Verification items for this drawing (mm, ordinates from the low corner). A direction names the side the tool comes from. Round coordinates to 2 decimals unless told otherwise and drop trailing zeros. Loops run counter-clockwise (first coordinate to the right, second up) from the corner with the lowest first, then second, coordinate; pieces in that order, holes last. Notation, with made-up numbers: M 77.5,59 L 89.5,59 A31 ccw 89.5,88 Z; hole C 77.5,-17 d3. An arc over 180 degrees is marked long. Use one line per item in the form item = value. Start each with the question number.
1. Cross-section at B-B (z = 46). Record the boundary of the cut face in (x, y), then the cut area to 3 significant figures.
2. Set-up check for the marked faces 1 and 2: record each of +Z, -Z, +X, -X, +Y, -Y from which the full face is reachable in a straight line by a thin tool's end or side.
3. Cross-section at A-A (x = 25). Record the boundary of the cut face in (y, z), then the cut area to 3 significant figures.
4. Go/stop test with flat-tipped pins: pin 1 (6 mm diameter, centred on x = 5, z = 43.5, fed in from -Y); pin 2 (1 mm diameter, centred on x = 25, y = 18.5, fed in from +Z); pin 3 (2 mm diameter, centred on x = 42.5, z = 20.5, fed in from +Y). Record where each tip stops, or that it passes through.
5. Material ranges on line 1 (Z direction, x = 35, y = 23); line 2 (Z direction, x = 38.5, y = 8), recorded low to high.
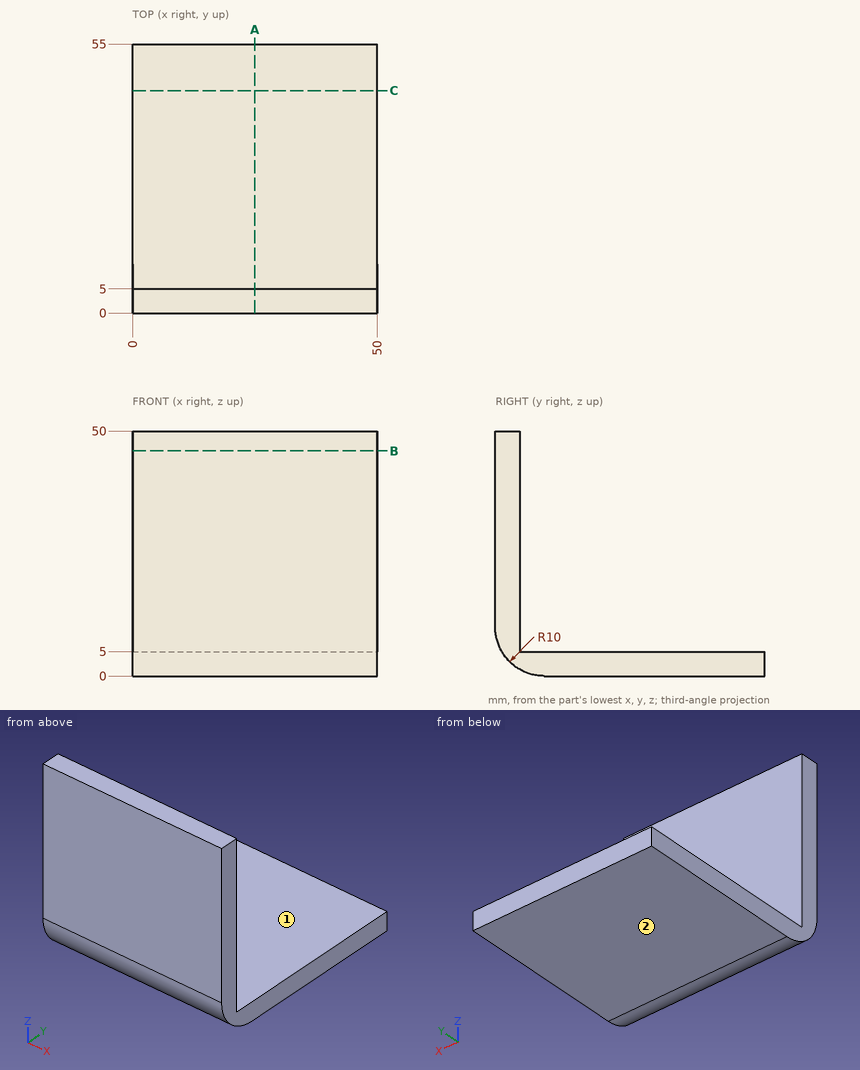
Reported:
q1.outline = M 0,0 L 50,0 L 50,5 L 0,5 Z
q1.area = 250 mm²
q2.face_1 = +Z, +X, -X, +Y
q2.face_2 = -Z, +X, -X, +Y, -Y
q3.outline = M 0,10 A10 ccw 10,0 L 55,0 L 55,5 L 5,5 L 5,50 L 0,50 Z
q3.area = 479 mm²
q4.pin_1 = 0
q4.pin_2 = 5
q4.pin_3 = 5
q5.line_1 = 0 to 5
q5.line_2 = 0.2 to 5
